from build123d import *

# Parameters (mm, degrees)
F0_W      = 196.0822343826
F0_H      = 109.9328920245
F1_DEPTH  = 62.8
F2_W      = 168.0704802275
F2_H      = 109.4043701887
F3_DEPTH  = 95
F4_R      = 6.9163922732
F5_DEPTH  = 8.9
F6_W      = 18.5355395079
F6_H      = 9.5271170139
F7_DEPTH  = 22
F8_W      = 6.9370792508
F8_H      = 18.5355395079
F9_DEPTH  = 14.1
F10_R     = 5
F11_R     = 6.8989817164
F11_R_2   = 6.9010656104
F12_DEPTH = 9.9


with BuildPart() as f1:
    # F0 (on Front) → F1 (new body, symmetric)
    with BuildSketch(Plane.XZ):
        Rectangle(F0_W, F0_H)
    extrude(amount=F1_DEPTH, both=True)

    # F2 (on face) → F3 (cut)
    with BuildSketch(Plane.XY.offset(54.9664460123)):
        with Locations((5.2852407098, -0.2642609179)):
            Rectangle(F2_W, F2_H)
    extrude(amount=-F3_DEPTH, mode=Mode.SUBTRACT)

    # F4 (on face) → F5 (cut)
    with BuildSketch(Plane.XY.offset(-40.0335539877)):
        with Locations((-64.4798651338, 0)):
            Circle(F4_R)
    extrude(amount=-F5_DEPTH, mode=Mode.SUBTRACT)

    # F6 (on face) → F7 (join)
    with BuildSketch(Plane.YZ.offset(-78.749999404)):
        with Locations((0, 38.6865362525)):
            Rectangle(F6_W, F6_H)
    extrude(amount=F7_DEPTH)

    # F8 (on face) → F9 (join)
    with BuildSketch(Plane.XY.offset(43.4500947595)):
        with Locations((-60.2185390294, 0)):
            Rectangle(F8_W, F8_H)
    extrude(amount=-F9_DEPTH)

    # F10
    f10_edges = [f1.edges().sort_by_distance(p)[0] for p in [
        (5.285241, -54.966446, 54.966446),
        (89.320481, -54.966446, 7.466446),
        (5.285241, -54.966446, -40.033554),
        (-67.749999, 9.26777, 43.450095),
        (-67.749999, -9.26777, 43.450095),
        (-56.749999, 0, 43.450095),
        (-60.218539, 9.26777, 29.350095),
        (-56.749999, -9.26777, 36.400095),
        (-78.749999, -0.264261, 54.966446),
        (5.285241, 54.437924, 54.966446),
        (-78.749999, -0.264261, -40.033554),
        (5.285241, 54.437924, -40.033554),
        (89.320481, -0.264261, -40.033554),
        (-56.749999, 9.26777, 36.400095),
        (89.320481, -0.264261, 54.966446),
    ]]
    fillet(f10_edges, radius=F10_R)

    # F11 (on face) → F12 (join)
    with BuildSketch(Plane.YZ.offset(-78.749999404)):
        with Locations((-24.7665680945, 33.9229777455)):
            Circle(F11_R)
        with Locations((23.0645500124, 33.9229777455)):
            Circle(F11_R_2)
    extrude(amount=F12_DEPTH)


solid = f1.part
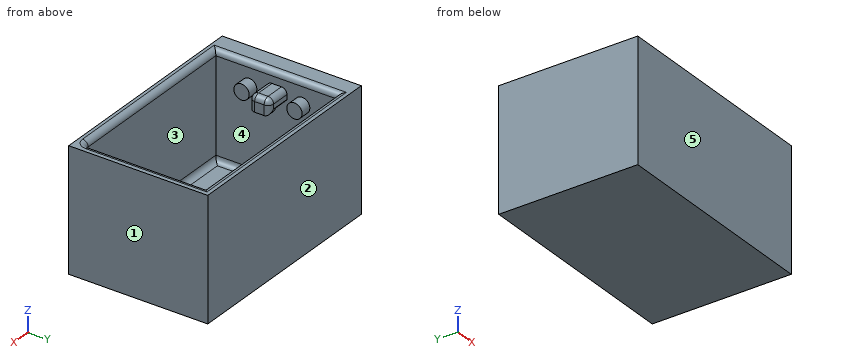
The listing builds one solid part. Answer for the finished solid, in the listing's coordinates (mm). Face numbers are marked on the shaded views. A direction names the side the tool comes from. Round coordinates to 2 decimals unless told otherwise and drop trailing zeros. Loops run counter-clockwise (first coordinate to the right, second up) from the corner with the lowest first, then second, coordinate; pieces in that order, holes last. Notation, with made-up numbers: M -31.5,53 L -23.5,53 A21 ccw -23.5,78 Z; hole C 46.25,63.5 d2. An arc over 180 degrees is marked long. Write each question's results on one line, items separated by ' | '. Start each with the question number.
1) Each of these flat-tipped pins is pushed along its axis until it touches: pin 1 (8 mm diameter, centred on x = 60.5, y = 13, fed in from +Z); pin 2 (22 mm diameter, centred on x = -64.48, y = 0, fed in from +Z). Where does it stop, or does it pass through?
2) Straight lines are drawn through the part: probe 1 along Y at (x, z) = (-22.5, 1.5); probe 2 along X at (y, z) = (-19, -25); probe 3 along Z at (x, y) = (32.5, 3.5). For each, find the intervals that lie inside material, in ascending order.
3) Which of the six approach directions +Z, -Z, +X, -X, +Y, -Y give full straight-line access (tool end or side, diameter ignored) to the marked faces 4 and 5?
4) Find section C-C on x = 2. Write down the section's boundary in (y, z).
5) Find section D-D on y = 0. Write down the section's boundary in (x, z).
6) Find section B-B on y = -37. Write down the section's boundary in (x, z), plus the area to 3 significant figures.
7) Determine the mould class of the marked faces 1, 2 and 3 for opening direction X: pulls with the +X half, pulls with the -X half, needs draft (parallel to the pull), parting line crosses it, or undercut.
8) Find section A-A on z = 5. Write down the section's boundary in (x, y), plus the area to 3 significant figures.
Final values:
1) pin 1: z = -40.03 | pin 2: z = 43.45
2) probe 1: -62.8 to -54.97, 54.44 to 62.8 | probe 2: -98.04 to -78.75, 89.32 to 98.04 | probe 3: -54.97 to -40.03
3) face 4: none | face 5: +Z, -Z, +X, -X, -Y
4) outline: M -62.8,-54.97 L 62.8,-54.97 L 62.8,54.97 L 59.44,54.97 A5 ccw 54.44,49.97 L 54.44,-35.03 A5 cw 49.44,-40.03 L -49.97,-40.03 A5 cw -54.97,-35.03 L -54.97,49.97 A5 ccw -59.97,54.97 L -62.8,54.97 Z
5) outline: M -98.04,-54.97 L 98.04,-54.97 L 98.04,54.97 L 94.32,54.97 A5 ccw 89.32,49.97 L 89.32,-35.03 A5 cw 84.32,-40.03 L -57.56,-40.03 L -57.56,-48.93 L -71.4,-48.93 L -71.4,-40.03 L -73.75,-40.03 A5 cw -78.75,-35.03 L -78.75,33.92 L -63.69,33.92 L -63.69,29.35 L -56.75,29.35 L -56.75,38.45 A5 ccw -61.75,43.45 L -78.75,43.45 L -78.75,49.97 A5 ccw -83.75,54.97 L -98.04,54.97 Z
6) outline: M -98.04,-54.97 L 98.04,-54.97 L 98.04,54.97 L 94.32,54.97 A5 ccw 89.32,49.97 L 89.32,-35.03 A5 cw 84.32,-40.03 L -73.75,-40.03 A5 cw -78.75,-35.03 L -78.75,49.97 A5 ccw -83.75,54.97 L -98.04,54.97 Z | area: 5,590 mm²
7) face 1: pulls with the +X half | face 2: needs draft | face 3: undercut
8) outline: M -98.04,-62.8 L 98.04,-62.8 L 98.04,62.8 L -98.04,62.8 Z; hole M -78.75,-54.97 L 84.32,-54.97 A5 ccw 89.32,-49.97 L 89.32,54.44 L -78.75,54.44 Z | area: 6,250 mm²
